Check sheet for the modelled part. Datum: model origin and axes. Units: mm. A direction names the side the tool comes from. Coordinates: 2 decimals unless noted, no trailing zeros. Write each loop counter-clockwise with the first axis right and the second up, starting at its lowest first coordinate (ties: lowest second). Pieces come first, ordered by that corner, then holes. Notation, with made-up numbers: (-22.5, 80) -> (5.5, 80) arc R12 cw to (5.5, 88) -> close; hole circle Ø1 at (-29, 9.5). An arc over 180 degrees is marked (long way). One line per item, written item: value. Start each with the question number.
1) Scan lines: line 1 along X through (y, z) = (-5, 103); line 2 along Z through (x, y) = (86, -2.75); line 3 along X through (y, z) = (-3.75, 96.5). Record each from-to range of solid material in increasing order. Write a range as [from, to].
2) Draft check along Z on faces 4 (the flat face through (115, -7.55, 105)), 5 (the cylindrical face through (95.5, -3.7, 102.9)), 6 (the flat face through (89, -1, 0)). Enter one of: +Z half, -Z half, draft (parallel to the pull), parting line (faces both ways), or undercut.
3) Gauge pin test, flat ends, axial feed: P1, Ø4, axis at x = 72, z = 94, coming from the -Y side; P2, Ø2.5, axis at x = 20.5, y = -4, coming from the -Z side. Record the tip position at first contact, or that the pin passes through.
4) Sectioned sample at B-B on z = 112. Enter the section's corners in (x, y), plus the area to 3 significant figures.
5) Sectioned sample at C-C on x = 44. Enter the section's corners in (y, z), plus the area to 3 significant figures.
6) Set-up check for faces 1 (the flat face through (111, 0, 103)), 2 (the flat face through (33, -4, 90.1)), 3 (the flat face through (73, -4, 129.12)): record each of +Z, -Z, +X, -X, +Y, -Y from which the full face is reachable in a straight line by a thin tool's end or side.
7) Sectioned sample at A-A on x = 113.5. Enter the section's corners in (y, z), plus the area to 3 significant figures.
```python
from build123d import *

# Parameters (mm, degrees)
SKETCH3_W           = 149
SKETCH3_H           = 141.12
BOSS_EXTRUDE1_DEPTH = 4
SKETCH5_W           = 67
SKETCH5_H           = 30.2
SKETCH5_H_2         = 36.8
BOSS_EXTRUDE2_DEPTH = 11.55
FILLET1_R           = 2
SKETCH6_W           = 149
SKETCH6_H           = 12
BOSS_EXTRUDE3_DEPTH = 7.5
FILLET2_R           = 2


with BuildPart() as part:
    # Sketch3 → Boss-Extrude1 (new body)
    with BuildSketch(Plane(origin=(0, 0, 0), x_dir=(1, 0, 0), z_dir=(0, 1, 0))):
        with Locations((74.5, -70.56)):
            Rectangle(SKETCH3_W, SKETCH3_H)
    extrude(amount=BOSS_EXTRUDE1_DEPTH)

    # Sketch5 → Boss-Extrude2 (add)
    # profile 1 of 6: a face of its own
    with BuildSketch(Plane(origin=(0, 4, 0), x_dir=(1, 0, 0), z_dir=(0, 1, 0))):
        with Locations((33.5, -25)):
            Rectangle(SKETCH5_W, SKETCH5_H)
        with BuildLine():
            ThreePointArc((12.85, -27.8), (11.05, -26), (12.85, -24.2))
            Line((12.85, -24.2), (40.15, -24.2))
            ThreePointArc((40.15, -24.2), (41.95, -26), (40.15, -27.8))
            Line((40.15, -27.8), (12.85, -27.8))
        make_face(mode=Mode.SUBTRACT)
    # profile 2 of 6: a face of its own
    with BuildSketch(Plane(origin=(0, 4, 0), x_dir=(1, 0, 0), z_dir=(0, 1, 0))):
        with Locations((115.5, -18.4)):
            Rectangle(SKETCH5_W, SKETCH5_H_2)
        with BuildLine():
            ThreePointArc((97.3, -24.5), (95.5, -22.7), (97.3, -20.9))
            Line((97.3, -20.9), (124.6, -20.9))
            ThreePointArc((124.6, -20.9), (126.4, -22.7), (124.6, -24.5))
            Line((124.6, -24.5), (97.3, -24.5))
        make_face(mode=Mode.SUBTRACT)
    # profile 3 of 6: a face of its own
    with BuildSketch(Plane(origin=(0, 4, 0), x_dir=(1, 0, 0), z_dir=(0, 1, 0))):
        with Locations((33.5, -65.1)):
            Rectangle(SKETCH5_W, SKETCH5_H)
        with BuildLine():
            ThreePointArc((12.85, -67.9), (11.05, -66.1), (12.85, -64.3))
            Line((12.85, -64.3), (40.15, -64.3))
            ThreePointArc((40.15, -64.3), (41.95, -66.1), (40.15, -67.9))
            Line((40.15, -67.9), (12.85, -67.9))
        make_face(mode=Mode.SUBTRACT)
    # profile 4 of 6: a face of its own
    with BuildSketch(Plane(origin=(0, 4, 0), x_dir=(1, 0, 0), z_dir=(0, 1, 0))):
        with Locations((115.5, -61.8)):
            Rectangle(SKETCH5_W, SKETCH5_H)
        with BuildLine():
            ThreePointArc((97.3, -64.6), (95.5, -62.8), (97.3, -61))
            Line((97.3, -61), (124.6, -61))
            ThreePointArc((124.6, -61), (126.4, -62.8), (124.6, -64.6))
            Line((124.6, -64.6), (97.3, -64.6))
        make_face(mode=Mode.SUBTRACT)
    # profile 5 of 6: a face of its own
    with BuildSketch(Plane(origin=(0, 4, 0), x_dir=(1, 0, 0), z_dir=(0, 1, 0))):
        with Locations((33.5, -105.2)):
            Rectangle(SKETCH5_W, SKETCH5_H)
        with BuildLine():
            ThreePointArc((12.85, -108), (11.05, -106.2), (12.85, -104.4))
            Line((12.85, -104.4), (40.15, -104.4))
            ThreePointArc((40.15, -104.4), (41.95, -106.2), (40.15, -108))
            Line((40.15, -108), (12.85, -108))
        make_face(mode=Mode.SUBTRACT)
    # profile 6 of 6: a face of its own
    with BuildSketch(Plane(origin=(0, 4, 0), x_dir=(1, 0, 0), z_dir=(0, 1, 0))):
        with Locations((115.5, -101.9)):
            Rectangle(SKETCH5_W, SKETCH5_H)
        with BuildLine():
            ThreePointArc((97.3, -104.7), (95.5, -102.9), (97.3, -101.1))
            Line((97.3, -101.1), (124.6, -101.1))
            ThreePointArc((124.6, -101.1), (126.4, -102.9), (124.6, -104.7))
            Line((124.6, -104.7), (97.3, -104.7))
        make_face(mode=Mode.SUBTRACT)
    extrude(amount=-BOSS_EXTRUDE2_DEPTH)

    # Fillet1
    fillet1_edges = [part.edges().sort_by_distance(p)[0] for p in [
        (67, -3.775, 50),
        (67, -3.775, 80.2),
        (0, -3.775, 80.2),
        (0, -3.775, 50),
        (82, -3.775, 46.7),
        (149, -3.775, 46.7),
        (149, -3.775, 76.9),
        (82, -3.775, 76.9),
        (67, -3.775, 90.1),
        (67, -3.775, 120.3),
        (0, -3.775, 120.3),
        (0, -3.775, 90.1),
        (82, -3.775, 86.8),
        (149, -3.775, 86.8),
        (149, -3.775, 117),
        (82, -3.775, 117),
        (67, -3.775, 9.9),
        (67, -3.775, 40.1),
        (0, -3.775, 40.1),
        (0, -3.775, 9.9),
        (82, -3.775, 0),
        (149, -3.775, 36.8),
        (82, -3.775, 36.8),
        (149, -1.775, 0),
    ]]
    fillet(fillet1_edges, radius=FILLET1_R)

    # Sketch6 → Boss-Extrude3 (add)
    with BuildSketch(Plane.XZ):
        with Locations((74.5, 135.12)):
            Rectangle(SKETCH6_W, SKETCH6_H)
    extrude(amount=BOSS_EXTRUDE3_DEPTH)

    # Fillet2
    fillet2_edges = [part.edges().sort_by_distance(p)[0] for p in [
        (0, -3.75, 129.12),
        (149, -3.75, 129.12),
    ]]
    fillet(fillet2_edges, radius=FILLET2_R)


solid = part.part
```
Answers:
1. line 1: x = [0, 67], [82, 95.5], [126.4, 149]
1. line 2: z = [0, 36.8], [46.7, 76.9], [86.8, 117], [129.12, 141.12]
1. line 3: x = [0, 67], [82, 149]
2. face 4: draft
2. face 5: undercut
2. face 6: -Z half
3. P1: stops at y = 0
3. P2: stops at z = 9.9
4. outline: (0, -7.55) -> (67, -7.55) -> (67, 0) -> (82, 0) -> (82, -7.55) -> (149, -7.55) -> (149, 4) -> (0, 4) -> close
4. area: 1,610 mm2
5. outline: (-7.55, 9.9) -> (0, 9.9) -> (0, 0) -> (4, 0) -> (4, 141.12) -> (-7.5, 141.12) -> (-7.5, 129.12) -> (0, 129.12) -> (0, 120.3) -> (-7.55, 120.3) -> (-7.55, 90.1) -> (0, 90.1) -> (0, 80.2) -> (-7.55, 80.2) -> (-7.55, 50) -> (0, 50) -> (0, 40.1) -> (-7.55, 40.1) -> close
5. area: 1,340 mm2
6. face 1: -Y
6. face 2: -X, -Y
6. face 3: +X, -X, -Y
7. outline: (-7.55, 0) -> (4, 0) -> (4, 141.12) -> (-7.5, 141.12) -> (-7.5, 129.12) -> (0, 129.12) -> (0, 117) -> (-7.55, 117) -> (-7.55, 104.7) -> (0, 104.7) -> (0, 101.1) -> (-7.55, 101.1) -> (-7.55, 86.8) -> (0, 86.8) -> (0, 76.9) -> (-7.55, 76.9) -> (-7.55, 64.6) -> (0, 64.6) -> (0, 61) -> (-7.55, 61) -> (-7.55, 46.7) -> (0, 46.7) -> (0, 36.8) -> (-7.55, 36.8) -> (-7.55, 24.5) -> (0, 24.5) -> (0, 20.9) -> (-7.55, 20.9) -> close
7. area: 1,310 mm2
